Model file for the job. Use its own axes, mm. Coordinates: 2 decimals unless noted, no trailing zeros. Write each loop counter-clockwise with the first axis right and the second up, starting at its lowest first coordinate (ties: lowest second). Pieces come first, ordered by that corner, then holes. Notation, with made-up numbers: M -15.5,61 L -5.5,61 A6 ccw -5.5,69 Z; hole C -7.5,-14 d11. An arc over 180 degrees is marked long. One line per question, with ' | ' between items. Start each with the question number.
(1) Cut at D-D (z = -11). Write the cut outline in (x, y).
(2) Cut at B-B (y = 0.35). Count the separate pieces of the cut face and the enclosed holes in it, plus the area to 3 significant figures.
(3) Flat gauge pins, fed straight in: pin 1 Ø1 at (x, y) = (-7, 1) entering from +Z; pin 2 Ø1 at (x, y) = (-21.5, 1) entering from +Z; pin 3 Ø0.9 at (x, y) = (6, 1.5) entering from -Z. Where does each tip first touch, or does it go through?
(4) Cut at A-A (x = -22.5). Write the cut outline in (y, z), plus the area to 3 significant figures.
(5) Cut at C-C (x = 19.5). Write the cut outline in (y, z).
(6) Wall check: probe 1 along X at (y, z) = (0.4, -23); probe 2 along X at (y, z) = (1.25, -5); probe 3 along X at (y, z) = (1.25, -1.5). Give the ranges that are in metal, low to high.
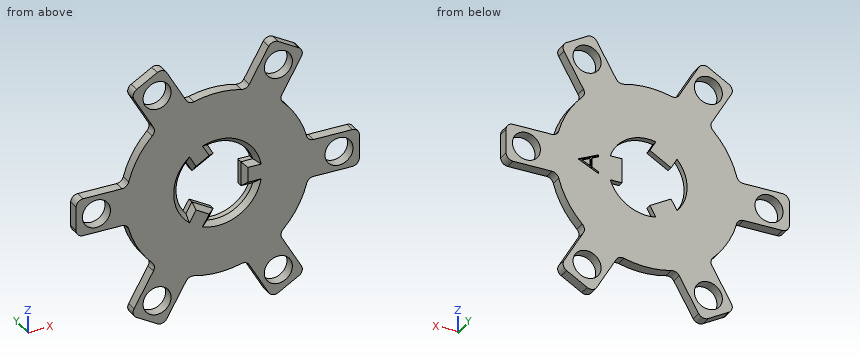
from build123d import *

# Parameters (mm, degrees)
SKETCH1_R           = 2.4
BOSS_EXTRUDE1_DEPTH = 1.8
FILLET11_R          = 1.2
CUT_EXTRUDE3_DEPTH  = 0.4
CUT_EXTRUDE4_DEPTH  = 2.5
CHAMFER1_SIZE       = 0.8
SCALE1_SCALE        = 1.15


with BuildPart() as part:
    # Sketch1 → Boss-Extrude1 (new body)
    with BuildSketch(Plane(origin=(0, 0, 0), x_dir=(1, 0, 0), z_dir=(0, 1, 0))):
        with BuildLine():
            Line((4.929751496, -15.011247456), (9.329383596, -22.631633787))
            Line((9.329383596, -22.631633787), (14.934877991, -19.395300089))
            Line((14.934877991, -19.395300089), (10.535245891, -11.774913758))
            ThreePointArc((10.535245891, -11.774913758), (13.68320138, -7.9), (15.464997388, -3.236333698))
            Line((15.464997388, -3.236333698), (24.264261587, -3.236333698))
            Line((24.264261587, -3.236333698), (24.264261587, 3.236333698))
            Line((24.264261587, 3.236333698), (15.464997388, 3.236333698))
            ThreePointArc((15.464997388, 3.236333698), (13.68320138, 7.9), (10.535245891, 11.774913758))
            Line((10.535245891, 11.774913758), (14.934877991, 19.395300089))
            Line((14.934877991, 19.395300089), (9.329383596, 22.631633787))
            Line((9.329383596, 22.631633787), (4.929751496, 15.011247456))
            ThreePointArc((4.929751496, 15.011247456), (0, 15.8), (-4.929751496, 15.011247456))
            Line((-4.929751496, 15.011247456), (-9.329383596, 22.631633787))
            Line((-9.329383596, 22.631633787), (-14.934877991, 19.395300089))
            Line((-14.934877991, 19.395300089), (-10.535245891, 11.774913758))
            ThreePointArc((-10.535245891, 11.774913758), (-13.68320138, 7.9), (-15.464997388, 3.236333698))
            Line((-15.464997388, 3.236333698), (-24.264261587, 3.236333698))
            Line((-24.264261587, 3.236333698), (-24.264261587, -3.236333698))
            Line((-24.264261587, -3.236333698), (-15.464997388, -3.236333698))
            ThreePointArc((-15.464997388, -3.236333698), (-13.68320138, -7.9), (-10.535245891, -11.774913758))
            Line((-10.535245891, -11.774913758), (-14.934877991, -19.395300089))
            Line((-14.934877991, -19.395300089), (-9.329383596, -22.631633787))
            Line((-9.329383596, -22.631633787), (-4.929751496, -15.011247456))
            ThreePointArc((-4.929751496, -15.011247456), (0, -15.8), (4.929751496, -15.011247456))
        make_face()
        with Locations((20.784609691, 0)):
            Circle(SKETCH1_R, mode=Mode.SUBTRACT)
        with Locations((10.392304845, -18)):
            Circle(SKETCH1_R, mode=Mode.SUBTRACT)
        with Locations((-10.392304845, -18)):
            Circle(SKETCH1_R, mode=Mode.SUBTRACT)
        with Locations((-20.784609691, 0)):
            Circle(SKETCH1_R, mode=Mode.SUBTRACT)
        with Locations((-10.392304845, 18)):
            Circle(SKETCH1_R, mode=Mode.SUBTRACT)
        with Locations((10.392304845, 18)):
            Circle(SKETCH1_R, mode=Mode.SUBTRACT)
    extrude(amount=BOSS_EXTRUDE1_DEPTH)

    # Fillet11
    fillet11_edges = [part.edges().sort_by_distance(p)[0] for p in [
        (24.264261587, 0.9, 3.236333698),
        (15.464997388, 0.9, 3.236333698),
        (10.535245891, 0.9, 11.774913758),
        (14.934877991, 0.9, 19.395300089),
        (9.329383596, 0.9, 22.631633787),
        (4.929751496, 0.9, 15.011247456),
        (-4.929751496, 0.9, 15.011247456),
        (-9.329383596, 0.9, 22.631633787),
        (-14.934877991, 0.9, 19.395300089),
        (-10.535245891, 0.9, 11.774913758),
        (-15.464997388, 0.9, 3.236333698),
        (-24.264261587, 0.9, 3.236333698),
        (-24.264261587, 0.9, -3.236333698),
        (-15.464997388, 0.9, -3.236333698),
        (-10.535245891, 0.9, -11.774913758),
        (-14.934877991, 0.9, -19.395300089),
        (-9.329383596, 0.9, -22.631633787),
        (-4.929751496, 0.9, -15.011247456),
        (4.929751496, 0.9, -15.011247456),
        (9.329383596, 0.9, -22.631633787),
        (14.934877991, 0.9, -19.395300089),
        (10.535245891, 0.9, -11.774913758),
        (15.464997388, 0.9, -3.236333698),
        (24.264261587, 0.9, -3.236333698),
    ]]
    fillet(fillet11_edges, radius=FILLET11_R)

    # Sketch10 → Cut-Extrude3 (cut)
    with BuildSketch(Plane(origin=(0, 1.8, 0), x_dir=(1, 0, 0), z_dir=(0, 1, 0))):
        Polygon((11.897175645, -0.131244585), (8.397175645, -1.7466292), (8.397175645, -1.405182886), (9.518970517, -0.887755001), (9.518970517, 0.698883621), (8.397175645, 1.231035063), (8.397175645, 1.573883621), (11.897175645, -0.08637279), align=None)
        Polygon((11.214984138, -0.105303078), (9.877944876, 0.528511024), (9.877944876, -0.722290258), align=None, mode=Mode.SUBTRACT)
    extrude(amount=-CUT_EXTRUDE3_DEPTH, mode=Mode.SUBTRACT)

    # Sketch11 → Cut-Extrude4 (cut, symmetric)
    with BuildSketch(Plane(origin=(0, 0, 0), x_dir=(1, 0, 0), z_dir=(0, 1, 0))):
        with BuildLine():
            Line((-0.367543966, -4.836604823), (-4.004850662, -2.736604823))
            Line((-4.004850662, -2.736604823), (-5.026164065, -4.505571528))
            ThreePointArc((-5.026164065, -4.505571528), (-6.75, 0), (-5.026164065, 4.505571528))
            Line((-5.026164065, 4.505571528), (-4.004850662, 2.736604823))
            Line((-4.004850662, 2.736604823), (-0.367543966, 4.836604823))
            Line((-0.367543966, 4.836604823), (-1.388857369, 6.605571528))
            ThreePointArc((-1.388857369, 6.605571528), (3.375, 5.845671476), (6.415021434, 2.1))
            Line((6.415021434, 2.1), (4.372394628, 2.1))
            Line((4.372394628, 2.1), (4.372394628, -2.1))
            Line((4.372394628, -2.1), (6.415021434, -2.1))
            ThreePointArc((6.415021434, -2.1), (3.375, -5.845671476), (-1.388857369, -6.605571528))
            Line((-1.388857369, -6.605571528), (-0.367543966, -4.836604823))
        make_face()
    extrude(amount=CUT_EXTRUDE4_DEPTH, both=True, mode=Mode.SUBTRACT)

    # Chamfer1
    chamfer1_edges = [part.edges().sort_by_distance(p)[0] for p in [
        (5.393708031, 0, -2.1),
        (4.372394628, 0, 0),
        (5.393708031, 0, 2.1),
        (3.375, 0, 5.845671476),
        (-0.878200668, 0, 5.721088175),
        (-2.186197314, 0, 3.786604823),
        (-4.515507363, 0, 3.621088175),
        (-6.75, 0, 0),
        (-4.515507363, 0, -3.621088175),
        (-2.186197314, 0, -3.786604823),
        (-0.878200668, 0, -5.721088175),
        (3.375, 0, -5.845671476),
    ]]
    chamfer(chamfer1_edges, length=CHAMFER1_SIZE)


with BuildPart() as part_1:
    # Scale1: scaled about (-0.006722783, 0.906799408, -6.4443e-05)
    add(part.part.scale(SCALE1_SCALE).moved(Location((0.001008417, -0.136019911, 9.666e-06))))


solid = part_1.part
Filled in:
1) outline: M -14.46,-0.14 L 14.46,-0.14 L 14.46,1.93 L -14.46,1.93 Z
2) separate pieces: 1 | enclosed holes: 7 | area: 1,150 mm²
3) pin 1: z = 20.44 | pin 2: z = 3.72 | pin 3: z = -18.61
4) outline: M -0.14,-3.72 L 1.93,-3.72 L 1.93,-2.38 L -0.14,-2.38 Z; M -0.14,2.38 L 1.93,2.38 L 1.93,3.72 L -0.14,3.72 Z | area: 5.56 mm²
5) outline: M -0.14,-3.72 L 1.93,-3.72 L 1.93,3.72 L -0.14,3.72 Z
6) probe 1: -15.97 to -13.48, -10.42 to -8.98, 8.98 to 10.43, 13.48 to 15.97 | probe 2: -17.47 to -5.94, -5.67 to -1.4, 5.94 to 17.47 | probe 3: -27.9 to -26.22, -21.58 to -7.62, 5.03 to 21.59, 26.22 to 27.9
